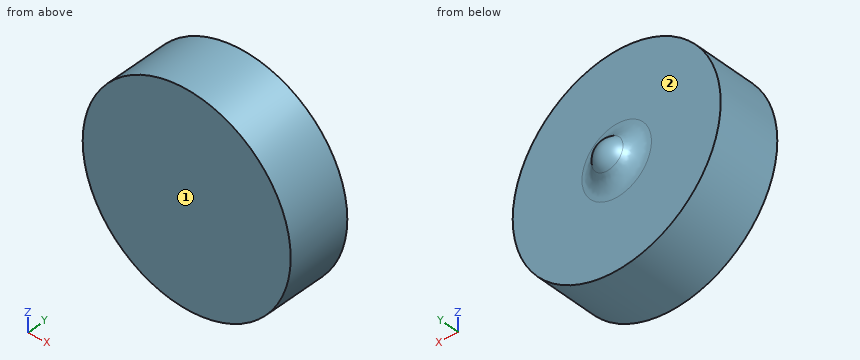
```python
from build123d import *

# Parameters (mm, degrees)
SKETCH_1_R      = 5
EXTRUDE_1_DEPTH = 3
FILLET_1_R      = 1.1


with BuildPart() as part:
    # 草图1 → 凸台-拉伸1 (new body)
    with BuildSketch(Plane(origin=(0, 0, 0), x_dir=(1, 0, 0), z_dir=(0, 1, 0))):
        Circle(SKETCH_1_R)
    extrude(amount=EXTRUDE_1_DEPTH)

    # 草图2 → 旋转1 (revolve)
    with BuildSketch(Plane.XY):
        with BuildLine():
            Line((0, 3.9), (0, 3))
            Line((0, 3), (0.9, 3))
            ThreePointArc((0.9, 3), (0.636396103, 3.636396103), (0, 3.9))
        make_face()
    revolve(axis=Axis((0, 0, 0), (0, 1, 0)))

    # 圆角1
    fillet_1_edges = [part.edges().sort_by_distance(p)[0] for p in [
        (-0.9, 3, 0),
    ]]
    fillet(fillet_1_edges, radius=FILLET_1_R)


solid = part.part
```
Geometry: final body of the model. Coordinates: model frame, mm. Face numbers are marked on the shaded views. A direction names the side the tool comes from. Give positions to 0.01 mm unless a question says otherwise; leave off trailing zeros. Loops run counter-clockwise (first coordinate to the right, second up) from the corner with the lowest first, then second, coordinate; pieces in that order, holes last. Notation, with made-up numbers: (61.5, -21) -> (71.5, -21) arc R19 cw to (71.5, 1) -> close; hole circle Ø6 at (89, 52.5). An arc over 180 degrees is marked (long way). Return JSON: item names as keys, results as strings.
Item 1: Section A-A, the plane z = 3. Output: boundary loops of the cut face in (x, y), plus the area to 3 significant figures.
Filled in:
{"outline": "(-4, 0) -> (4, 0) -> (4, 3) -> (-4, 3) -> close", "area": "24.0 mm^2"}
Item 2: Access query for the marked faces 1 and 2. Directions: +Z, -Z, +X, -X, +Y, -Y. A direction counts if a zero-diameter tool reaches every point of the face in a straight line with its end or side. Return the directions, or none.
Filled in:
{"face 1": "+Z, -Z, +X, -X, -Y", "face 2": "+Y"}
Item 3: Section C-C, the plane x = -3.75. Output: boundary loops of the cut face in (y, z).
Filled in:
{"outline": "(0, -3.31) -> (3, -3.31) -> (3, 3.31) -> (0, 3.31) -> close"}
Item 4: Line query: line 1 (Y direction, x = 0.5, z = -2.5); line 2 (X direction, y = 3.5, z = 0); line 3 (X direction, y = 0.8, z = 4.25). Output: solid intervals per line, ascending.
Filled in:
{"line 1": "0 to 3", "line 2": "-0.75 to 0.75", "line 3": "-2.63 to 2.63"}
Item 5: Section B-B, the plane y = 2.15. Output: boundary loops of the cut face in (x, z).
Filled in:
{"outline": "circle Ø10 at (0, 0)"}
Item 6: Pin query (flat end, axial travel): P1, Ø1.5, axis at x = -1, z = 3.5, coming from the +Y side; P2, Ø5, axis at x = 1.5, z = -2.5, coming from the -Y side; P3, Ø1, axis at y = 2, z = 4, coming from the -X side; P4, Ø2, axis at y = 3, z = 2, coming from the -X side. Return the tip coordinate at first contact, or that it passes through.
Filled in:
{"P1": "y = 3", "P2": "y = 0", "P3": "x = -3.57", "P4": "x = -4.9"}
